Could you check a few things on this drawing? It's one solid part, dimensions in mm from its lowest x, y, z. A direction names the side the tool comes from. Round coordinates to 2 decimals unless told otherwise and drop trailing zeros. Write each loop counter-clockwise with the first axis right and the second up, starting at its lowest first coordinate (ties: lowest second). Pieces come first, ordered by that corner, then holes. Notation, with made-up numbers: (43.5, -30) - (87.5, -30) arc R18 cw to (87.5, -1) - close; hole circle Ø4 at (-5, 66.25). An arc over 180 degrees is marked (long way). Put each result on its own line as item: value.
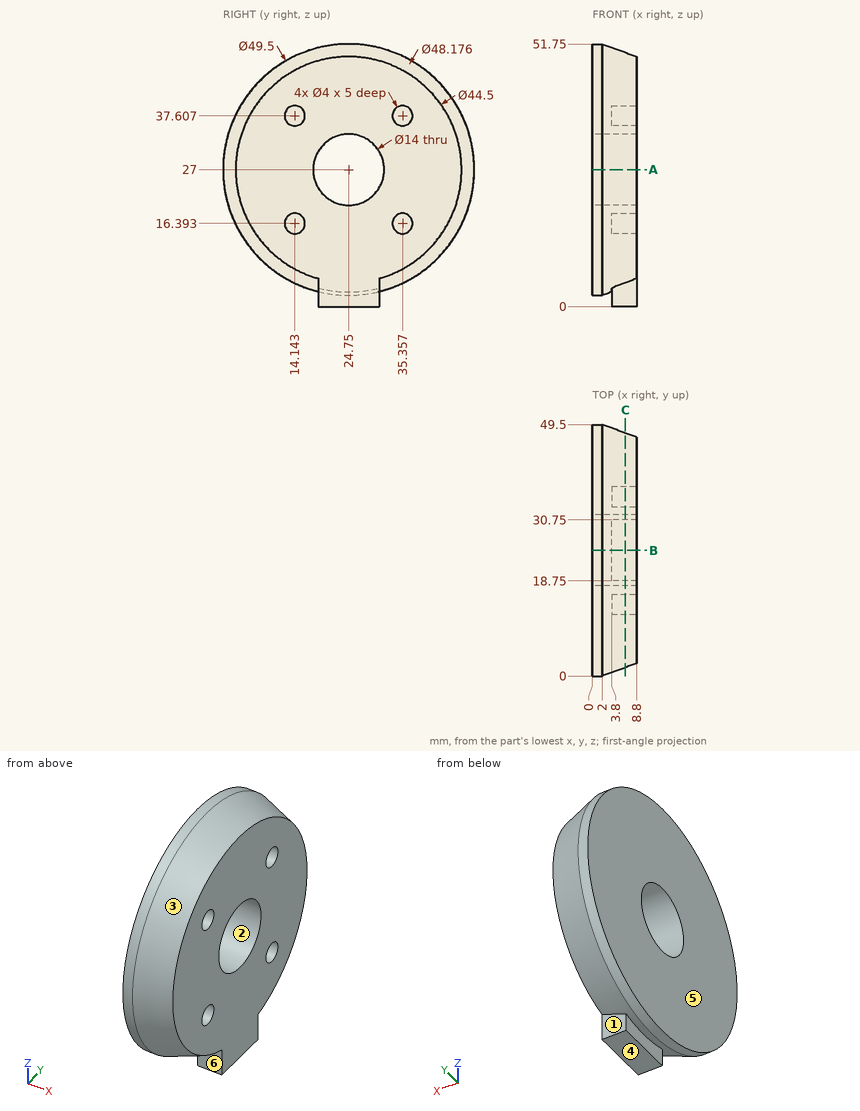
(1) Imagine slicing it at C-C, the plane x = 6.5. Give the number of separate pieces and of enclosed holes in the cut face, then the cut area to 3 significant figures.
Values found:
separate pieces: 1
enclosed holes: 5
area: 1,520 mm^2
(2) Imagine slicing it at A-A, the plane z = 27. List the corners of the cut face in (x, y) for me, then the cut area to 3 significant figures.
Values found:
outline: (0, 0) - (2, 0) - (8.8, 2.5) - (8.8, 17.75) - (0, 17.75) - close; (0, 31.75) - (8.8, 31.75) - (8.8, 47) - (2, 49.5) - (0, 49.5) - close
area: 295 mm^2
(3) For the marked faces 5 and 6, which set-ups out of +Z, -Z, +X, -X, +Y, -Y let a thin tool reach every point of the face, with its end or its side?
Values found:
face 5: +Z, -Z, -X, +Y, -Y
face 6: -Z, +X, -Y
(4) If we mould it in two halves opening along Z, with no side actions, what happens to the marked faces 1, 2, 3 and 4? For each: pulls with the +Z half, pulls with the -Z half, needs draft (parallel to the pull), parting line crosses it, or undercut.
Values found:
face 1: needs draft
face 2: undercut
face 3: parting line crosses it
face 4: pulls with the -Z half
(5) Imagine slicing it at B-B, the plane y = 24.75. List the corners of the cut face in (x, z) for me.
Values found:
outline: (0, 2.25) - (2, 2.25) - (3.8, 2.91) - (3.8, 0) - (8.8, 0) - (8.8, 20) - (0, 20) - close; (0, 34) - (8.8, 34) - (8.8, 49.25) - (2, 51.75) - (0, 51.75) - close
(6) Please list where these lines run through material, in increasing order: probe 1 along Z at (x, y) = (6, 14); probe 2 along Y at (x, z) = (7, 27); probe 3 along Z at (x, y) = (2, 23). Write a range as from..to.
Values found:
probe 1: z = 6.35..14.4, 18.39..35.61, 39.6..47.65
probe 2: y = 1.84..17.75, 31.75..47.66
probe 3: z = 2.31..20.22, 33.78..51.69
(7) I'm going to push flat-ended pins straight in: pin 1 (4 mm diameter, centred on x = 6.5, z = 2, fed in from -Y); pin 2 (1.2 mm diameter, centred on y = 36.5, z = 16.5, fed in from +X); pin 3 (1.5 mm diameter, centred on x = 5, z = 2, fed in from +Y). Where does each tip first touch, or does it pass through?
Values found:
pin 1: stops at y = 18.75
pin 2: stops at x = 3.8
pin 3: stops at y = 30.75
